Geometry: final body of the model. Coordinates: model frame, mm. Round coordinates to 2 decimals unless told otherwise and drop trailing zeros. Order: outer loops, then holes, each group sorted by start corner. A loop starts at its lowest first (then second) coordinate and runs counter-clockwise, first axis right, second up. Notation, with made-up numbers: (-31, 10) -> (7, 10) arc R11 ccw to (7, 16) -> close; hole circle Ø5 at (30, -25.75). An arc over 180 degrees is marked (long way). Put each result on its own line as item: value.
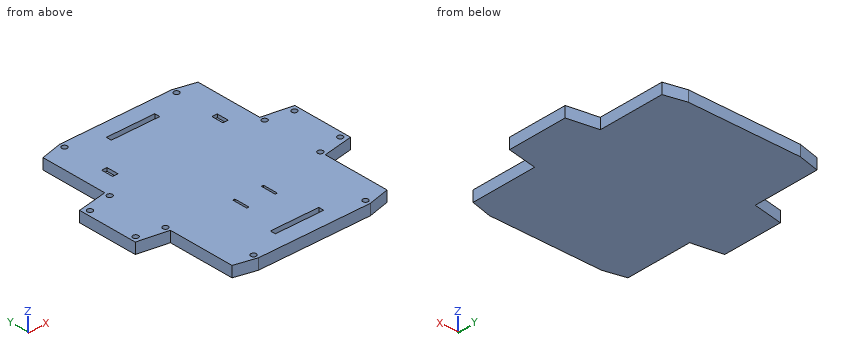
```python
from build123d import *

# Parameters (mm, degrees)
BOSS_EXTRUDE2_DEPTH     = 15
SKETCH2_W               = 3
SKETCH2_H               = 20
CUT_EXTRUDE2_DEPTH      = 10
SKETCH4_W               = 3
SKETCH4_H               = 20
BOSS_EXTRUDE5_DEPTH     = 10
CUT_EXTRUDE3_DEPTH      = 5
SKETCH6_R               = 2.5
CUT_EXTRUDE4_DEPTH      = 6
BOSS_EXTRUDE6_START     = -6
BOSS_EXTRUDE6_OUTLINE_R = 2.5
BOSS_EXTRUDE6_DEPTH     = 6
SKETCH8_R               = 2.5
CUT_EXTRUDE5_DEPTH      = 6
SKETCH9_W               = 2
SKETCH9_H               = 14
CUT_EXTRUDE6_DEPTH      = 3
SKETCH10_W              = 5
SKETCH10_H              = 11
CUT_EXTRUDE7_DEPTH      = 3
BOSS_EXTRUDE8_DEPTH     = 3
SKETCH12_W              = 5
SKETCH12_H              = 2
CUT_EXTRUDE8_DEPTH      = 3
SKETCH14_W              = 5
SKETCH14_H              = 7.25
BOSS_EXTRUDE9_DEPTH     = 3
SKETCH15_W              = 5
SKETCH15_H              = 7.25
CUT_EXTRUDE9_DEPTH      = 3
SKETCH16_W              = 5
SKETCH16_H              = 7.25
BOSS_EXTRUDE10_DEPTH    = 3
SKETCH17_W              = 5
SKETCH17_H              = 7.25
CUT_EXTRUDE10_DEPTH     = 3
SKETCH18_W              = 5
SKETCH18_H              = 7.25
BOSS_EXTRUDE11_DEPTH    = 3
SKETCH19_W              = 5
SKETCH19_H              = 7.25
CUT_EXTRUDE11_DEPTH     = 3
SKETCH20_W              = 5
SKETCH20_H              = 7.25
BOSS_EXTRUDE12_DEPTH    = 3
SKETCH21_W              = 5
SKETCH21_H              = 7.25
CUT_EXTRUDE12_DEPTH     = 3
SKETCH22_W              = 2
SKETCH22_H              = 7.25
CUT_EXTRUDE13_DEPTH     = 3
SKETCH23_W              = 2
SKETCH23_H              = 7.25
BOSS_EXTRUDE13_DEPTH    = 3
SKETCH24_W              = 45
SKETCH24_H              = 5
CUT_EXTRUDE14_DEPTH     = 5
SKETCH25_W              = 45
SKETCH25_H              = 5
BOSS_EXTRUDE17_DEPTH    = 5
SKETCH26_W              = 45
SKETCH26_H              = 5
CUT_EXTRUDE16_DEPTH     = 5


# Read off the part's stored shape, not the designer's step: Boss-Extrude6
with BuildPart() as part:
    # Sketch1 → Boss-Extrude2 (new body)
    with BuildSketch(Plane.XY):
        Polygon((-52, 100), (52, 100), (72, 95), (72, 33), (100, 28), (100, -28), (72, -33), (72, -95), (52, -100), (-52, -100), (-72, -95), (-72, -33), (-100, -28), (-100, 28), (-72, 33), (-72, 95.107401563), align=None)
    extrude(amount=BOSS_EXTRUDE2_DEPTH)

    # Sketch2 → Cut-Extrude2 (cut)
    with BuildSketch(Plane.XY.offset(15)):
        with Locations((-69.5, 80.352031484)):
            Rectangle(SKETCH2_W, SKETCH2_H)
        with Locations((-69.5, 43)):
            Rectangle(SKETCH2_W, SKETCH2_H)
    extrude(amount=-CUT_EXTRUDE2_DEPTH, mode=Mode.SUBTRACT)

    # Sketch4 → Boss-Extrude5 (add)
    with BuildSketch(Plane.XY.offset(15)):
        Polygon((-71, 90.352031484), (-68, 90.352031484), (-68, 70.352031484), (-69.5, 70.352031484), (-71, 70.352031484), align=None)
        with Locations((-69.5, 43)):
            Rectangle(SKETCH4_W, SKETCH4_H)
    extrude(amount=-BOSS_EXTRUDE5_DEPTH)

    # Sketch5 → Cut-Extrude3 (cut)
    with BuildSketch(Plane.XY.offset(15)):
        Polygon((-72, 95.107401563), (-72, 33), (-100, 28), (-100, -28), (-72, -33), (-72, -95), (-52, -100), (52, -100), (72, -95), (72, -33), (100, -28), (100, 28), (72, 33), (72, 95), (52, 100), (-52, 100), align=None)
    extrude(amount=-CUT_EXTRUDE3_DEPTH, mode=Mode.SUBTRACT)

    # Sketch6 → Cut-Extrude4 (cut)
    with BuildSketch(Plane.XY.offset(10)):
        with Locations((-95, -23)):
            Circle(SKETCH6_R)
        with Locations((-72, 28)):
            Circle(SKETCH6_R)
        with Locations((-72, -28)):
            Circle(SKETCH6_R)
        with Locations((-52, -95)):
            Circle(SKETCH6_R)
        with Locations((52, -95)):
            Circle(SKETCH6_R)
        with Locations((67, -28)):
            Circle(SKETCH6_R)
        with Locations((72, 28)):
            Circle(SKETCH6_R)
        with Locations((95, 23)):
            Circle(SKETCH6_R)
        with Locations((-52, 95.092484679)):
            Circle(SKETCH6_R)
        with Locations((52, 95.014916884)):
            Circle(SKETCH6_R)
        with Locations((95, -23)):
            Circle(SKETCH6_R)
        with Locations((-95, 23)):
            Circle(SKETCH6_R)
    extrude(amount=-CUT_EXTRUDE4_DEPTH, mode=Mode.SUBTRACT)

    # Boss-Extrude6 outline → Boss-Extrude6 (add)
    with BuildSketch(Plane.XY.offset(10).offset(BOSS_EXTRUDE6_START)):
        with Locations((67, -28)):
            Circle(BOSS_EXTRUDE6_OUTLINE_R)
    extrude(amount=BOSS_EXTRUDE6_DEPTH)

    # Sketch8 → Cut-Extrude5 (cut)
    with BuildSketch(Plane.XY.offset(10)):
        with Locations((-72, -28)):
            Circle(SKETCH8_R)
        with Locations(Location((72, -28, 0), (0, 0, 180))):
            Circle(SKETCH8_R)
    extrude(amount=-CUT_EXTRUDE5_DEPTH, mode=Mode.SUBTRACT)

    # Sketch9 → Cut-Extrude6 (cut)
    with BuildSketch(Plane.XY.offset(10)):
        with Locations((13.25, -33)):
            Rectangle(SKETCH9_W, SKETCH9_H)
        with Locations((-13.25, -33)):
            Rectangle(SKETCH9_W, SKETCH9_H)
    extrude(amount=-CUT_EXTRUDE6_DEPTH, mode=Mode.SUBTRACT)

    # Sketch10 → Cut-Extrude7 (cut)
    with BuildSketch(Plane.XY.offset(10)):
        with Locations((-51.19, 52.4)):
            Rectangle(SKETCH10_W, SKETCH10_H)
        with Locations((51.19, 52.4)):
            Rectangle(SKETCH10_W, SKETCH10_H)
    extrude(amount=-CUT_EXTRUDE7_DEPTH, mode=Mode.SUBTRACT)

    # Sketch11 → Boss-Extrude8 (add)
    with BuildSketch(Plane.XY.offset(10)):
        Polygon((-53.69, 55.9), (-48.69, 55.9), (-48.69, 57.549860814), (-48.69, 57.9), (-53.69, 57.9), align=None)
        Polygon((53.69, 57.9), (48.69, 57.9), (48.69, 55.9), (53.69, 55.9), (53.69, 57.549860814), align=None)
    extrude(amount=-BOSS_EXTRUDE8_DEPTH)

    # Sketch12 → Cut-Extrude8 (cut)
    with BuildSketch(Plane.XY.offset(10)):
        with Locations((-51.19, 45.9)):
            Rectangle(SKETCH12_W, SKETCH12_H)
        Polygon((53.69, 46.9), (48.69, 46.9), (48.69, 44.9), (53.69, 44.9), (53.69, 45.878343836), align=None)
    extrude(amount=-CUT_EXTRUDE8_DEPTH, mode=Mode.SUBTRACT)

    # Sketch14 → Boss-Extrude9 (add)
    with BuildSketch(Plane.XY.offset(10)):
        with Locations((-51.19, 48.525)):
            Rectangle(SKETCH14_W, SKETCH14_H)
    extrude(amount=-BOSS_EXTRUDE9_DEPTH)

    # Sketch15 → Cut-Extrude9 (cut)
    with BuildSketch(Plane.XY.offset(10)):
        with Locations((-51.19, 59.525)):
            Rectangle(SKETCH15_W, SKETCH15_H)
    extrude(amount=-CUT_EXTRUDE9_DEPTH, mode=Mode.SUBTRACT)

    # Sketch16 → Boss-Extrude10 (add)
    with BuildSketch(Plane.XY.offset(10)):
        with Locations((51.19, 48.525)):
            Rectangle(SKETCH16_W, SKETCH16_H)
    extrude(amount=-BOSS_EXTRUDE10_DEPTH)

    # Sketch17 → Cut-Extrude10 (cut)
    with BuildSketch(Plane.XY.offset(10)):
        with Locations((51.19, 59.525)):
            Rectangle(SKETCH17_W, SKETCH17_H)
    extrude(amount=-CUT_EXTRUDE10_DEPTH, mode=Mode.SUBTRACT)

    # Sketch18 → Boss-Extrude11 (add)
    with BuildSketch(Plane.XY.offset(10)):
        with Locations((-51.19, 59.525)):
            Rectangle(SKETCH18_W, SKETCH18_H)
    extrude(amount=-BOSS_EXTRUDE11_DEPTH)

    # Sketch19 → Cut-Extrude11 (cut)
    with BuildSketch(Plane.XY.offset(10)):
        with Locations((-51.19, 48.525)):
            Rectangle(SKETCH19_W, SKETCH19_H)
    extrude(amount=-CUT_EXTRUDE11_DEPTH, mode=Mode.SUBTRACT)

    # Sketch20 → Boss-Extrude12 (add)
    with BuildSketch(Plane.XY.offset(10)):
        with Locations((51.19, 59.525)):
            Rectangle(SKETCH20_W, SKETCH20_H)
    extrude(amount=-BOSS_EXTRUDE12_DEPTH)

    # Sketch21 → Cut-Extrude12 (cut)
    with BuildSketch(Plane.XY.offset(10)):
        with Locations((51.19, 48.525)):
            Rectangle(SKETCH21_W, SKETCH21_H)
    extrude(amount=-CUT_EXTRUDE12_DEPTH, mode=Mode.SUBTRACT)

    # Sketch22 → Cut-Extrude13 (cut)
    with BuildSketch(Plane.XY.offset(10)):
        with Locations((-13.25, -43.625)):
            Rectangle(SKETCH22_W, SKETCH22_H)
        with Locations((13.25, -43.625)):
            Rectangle(SKETCH22_W, SKETCH22_H)
    extrude(amount=-CUT_EXTRUDE13_DEPTH, mode=Mode.SUBTRACT)

    # Sketch23 → Boss-Extrude13 (add)
    with BuildSketch(Plane.XY.offset(10)):
        with Locations((-13.25, -29.625)):
            Rectangle(SKETCH23_W, SKETCH23_H)
        with Locations((13.25, -29.625)):
            Rectangle(SKETCH23_W, SKETCH23_H)
    extrude(amount=-BOSS_EXTRUDE13_DEPTH)

    # Sketch24 → Cut-Extrude14 (cut)
    with BuildSketch(Plane.XY.offset(10)):
        with Locations((0, 95.053700781)):
            Rectangle(SKETCH24_W, SKETCH24_H)
        with Locations((0, -95)):
            Rectangle(SKETCH24_W, SKETCH24_H)
    extrude(amount=-CUT_EXTRUDE14_DEPTH, mode=Mode.SUBTRACT)

    # Sketch25 → Boss-Extrude17 (add)
    with BuildSketch(Plane.XY.offset(5)):
        with Locations((0, 95.053700781)):
            Rectangle(SKETCH25_W, SKETCH25_H)
        with Locations((0, -95)):
            Rectangle(SKETCH25_W, SKETCH25_H)
    extrude(amount=BOSS_EXTRUDE17_DEPTH)

    # Sketch26 → Cut-Extrude16 (cut)
    with BuildSketch(Plane.XY.offset(10)):
        with Locations((0, -82.5)):
            Rectangle(SKETCH26_W, SKETCH26_H)
        with Locations((0, 82.5)):
            Rectangle(SKETCH26_W, SKETCH26_H)
    extrude(amount=-CUT_EXTRUDE16_DEPTH, mode=Mode.SUBTRACT)


solid = part.part
```
1. Cut plane D-D on x = 88. Return loops of the section in (y, z).
Ans:
outline: (-30.14, 0) -> (30.14, 0) -> (30.14, 10) -> (-30.14, 10) -> close
2. Cut plane A-A on y = 23. Return loops of the section in (x, z), and give its area (3 significant figures).
Ans:
outline: (-100, 0) -> (100, 0) -> (100, 10) -> (97.5, 10) -> (97.5, 4) -> (92.5, 4) -> (92.5, 10) -> (-92.5, 10) -> (-92.5, 4) -> (-97.5, 4) -> (-97.5, 10) -> (-100, 10) -> close
area: 1,940 mm²
3. Cut plane B-B on x = 3.5. Return loops of the section in (y, z), and give its area (3 significant figures).
Ans:
outline: (-100, 0) -> (100, 0) -> (100, 10) -> (85, 10) -> (85, 5) -> (80, 5) -> (80, 10) -> (-80, 10) -> (-80, 5) -> (-85, 5) -> (-85, 10) -> (-100, 10) -> close
area: 1,950 mm²
4. Contact query for flat-ended pins moving along their axis: P1, Ø1.5, axis at x = -94, y = -22.5, coming from the +Z side; P2, Ø3.5, axis at y = -38.5, z = 8, coming from the +X side; P3, Ø5.5, axis at y = 81.5, z = 8.5, coming from the -X side; P4, Ø3.5, axis at x = -52.5, z = 8.5, coming from the -Y side. Output: stop coordinate, or through.
Ans:
P1: z = 4
P2: x = 72
P3: x = -72
P4: y = -100
5. Material intervals for probe 1 along Y at (x, z) = (52, 6.65); probe 2 along X at (y, z) = (21.5, 5.75); probe 3 along Y at (x, z) = (50, 5.5), sorted ascending.
Ans:
probe 1: -100 to -97.5, -92.5 to 92.51, 97.51 to 100
probe 2: -100 to -97, -93 to 93, 97 to 100
probe 3: -100 to -96.5, -93.5 to 93.51, 96.51 to 100
6. Cut plane C-C on x = -65. Return loops of the section in (y, z), and give its area (3 significant figures).
Ans:
outline: (-96.75, 0) -> (96.82, 0) -> (96.82, 10) -> (-96.75, 10) -> close
area: 1,940 mm²
